Input: part model. Units: mm. Frame: model coordinates. Round coordinates to 2 decimals unless told otherwise and drop trailing zeros. Loops run counter-clockwise (first coordinate to the right, second up) from the corner with the lowest first, then second, coordinate; pieces in that order, holes last. Notation, with made-up numbers: M -14,-14.75 L 39,-14.75 A10 cw 39,4.25 Z; hole C 79,-4 d6. An arc over 180 degrees is marked long. Return JSON: item names as keys, results as strings. Group by question number.
1) Section C-C (y = -0.9). Output: boundary loops of the cut face in (x, z).
2) Section A-A (z = 0). Output: boundary loops of the cut face in (x, y), plus the area to 3 significant figures.
3) Section D-D (x = -9.5). Output: boundary loops of the cut face in (y, z), plus the area to 3 significant figures.
4) Contact query for flat-ended pins moving along their axis: P1, Ø1.5, axis at x = 9, y = -1, coming from the -Z side; P2, Ø1.4, axis at y = -2, z = 0.5, coming from the -X side; P3, Ø0.9, axis at x = 9, y = -1.5, coming from the +Z side. Output: stop coordinate, or through.
5) Material intervals for line 1 (Z direction, x = -0.5, y = -0.35); line 2 (Z direction, x = -5, y = -0.5) (3 decimals); line 3 (X direction, y = -2, z = 4.5), sorted ascending. Write a range as from..to.
6) Section B-B (x = 0). Output: boundary loops of the cut face in (y, z).
from build123d import *

# Parameters (mm, degrees)
F0_R     = 40
F0_R_2   = 8
F1_DEPTH = 3
F3_DEPTH = 3


with BuildPart() as f1:
    # F0 (on Front) → F1 (new body)
    with BuildSketch(Plane.XZ):
        Circle(F0_R)
        Circle(F0_R_2, mode=Mode.SUBTRACT)
    extrude(amount=F1_DEPTH)

    # F2 (on face) → F3 (cut, through all)
    with BuildSketch(Plane.XZ.offset(3)):
        with BuildLine():
            Line((10.8, -1.4), (10.8, 1.4))
            Line((10.8, 1.4), (7.876547, 1.4))
            ThreePointArc((7.876547, 1.4), (7.969077, 0.702716), (8, 0))
            ThreePointArc((8, 0), (7.969077, -0.702716), (7.876547, -1.4))
            Line((7.876547, -1.4), (10.8, -1.4))
        make_face()
    extrude(amount=-F3_DEPTH, mode=Mode.SUBTRACT)


solid = f1.part
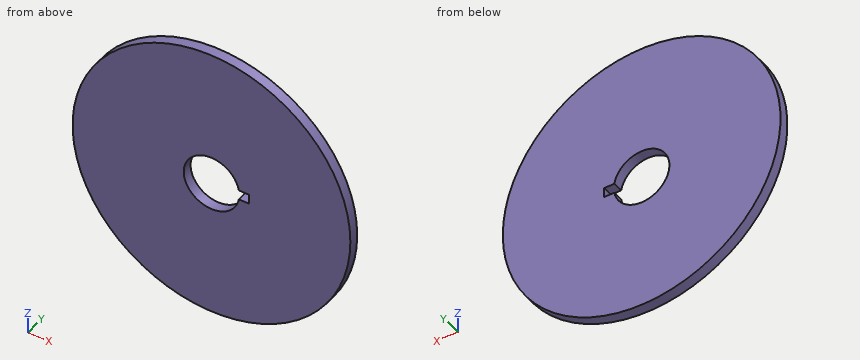
Returned:
{
 "1": {"outline": "C 0,0 d80; hole M 7.88,-1.4 L 10.8,-1.4 L 10.8,1.4 L 7.88,1.4 A8 ccw long Z"},
 "2": {"outline": "M -40,-3 L -8,-3 L -8,0 L -40,0 Z; M 10.8,-3 L 40,-3 L 40,0 L 10.8,0 Z", "area": "184 mm^2"},
 "3": {"outline": "M -3,-38.86 L 0,-38.86 L 0,38.86 L -3,38.86 Z", "area": "233 mm^2"},
 "4": {"P1": "stops at z = -39.14", "P2": "stops at x = -40", "P3": "stops at z = 39.08"},
 "5": {"line 1": "z = -40..-7.98, 7.98..40", "line 2": "z = -39.686..-6.245, 6.245..39.686", "line 3": "x = -39.75..-6.61, 6.61..39.75"},
 "6": {"outline": "M -3,-40 L 0,-40 L 0,-8 L -3,-8 Z; M -3,8 L 0,8 L 0,40 L -3,40 Z"}
}
